Part model, mm, in its own coordinate system. Face numbers are marked on the shaded views. A direction names the side the tool comes from. Round coordinates to 2 decimals unless told otherwise and drop trailing zeros. Write each loop counter-clockwise with the first axis right and the second up, starting at its lowest first coordinate (ties: lowest second). Pieces come first, ordered by that corner, then holes.
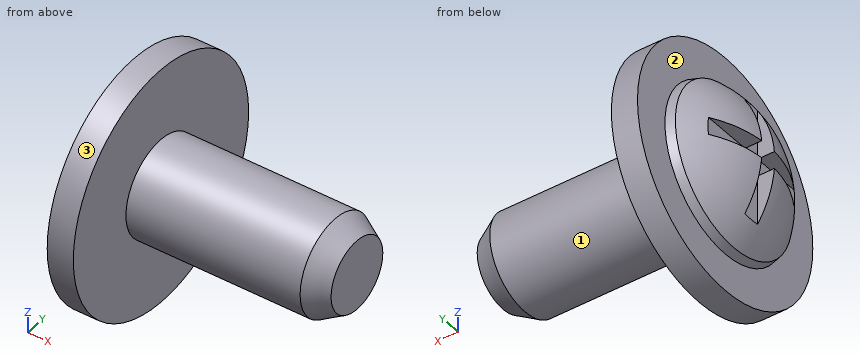
```python
from build123d import *

# Parameters (mm, degrees)
ESQUISSE2_W                  = 0.4
ESQUISSE2_H                  = 0.4
ENL_V_MAT_EXTRU_1_DEPTH      = 6.353036521
R_P_TITION_CIRCULAIRE1_COUNT = 2
R_P_TITION_CIRCULAIRE1_ANGLE = 90
ESQUISSE3_R                  = 2.75
BOSS_EXTRU_1_DEPTH           = 0.6


with BuildPart() as part:
    # Esquisse1 → Révolution1 (revolve)
    with BuildSketch(Plane.XY, mode=Mode.PRIVATE) as r_volution1_sk:
        with BuildLine():
            Line((0, 1.1), (0, 2.05))
            Line((0, 2.05), (-0.8, 1.835640646))
            ThreePointArc((-0.8, 1.835640646), (-1.391310546, 1.001196357), (-1.6, 0))
            Line((-1.6, 0), (4.5, 0))
            Line((4.5, 0), (4.5, 0.811324865))
            Line((4.5, 0.811324865), (4, 1.1))
            Line((4, 1.1), (0, 1.1))
        make_face()
    revolve(r_volution1_sk.sketch.rotate(Axis((-2.182265798, 0, 0), (1, 0, 0)), 90), axis=Axis((-2.182265798, 0, 0), (1, 0, 0)))

    # Esquisse2 → Enlèv. mat.-Extru.1 (cut, symmetric)
    with BuildSketch(Plane.XY):
        with Locations((-1.4, 0)):
            Rectangle(ESQUISSE2_W, ESQUISSE2_H)
    enl_v_mat_extru_1 = extrude(amount=ENL_V_MAT_EXTRU_1_DEPTH, both=True, mode=Mode.SUBTRACT)

    # Répétition circulaire1: Enlèv. mat.-Extru.1 ×2 about axis
    r_p_tition_circulaire1_axis = Axis((-2.182265798, 0, 0), (-1, 0, 0))
    for i in range(1, R_P_TITION_CIRCULAIRE1_COUNT):
        add(enl_v_mat_extru_1.rotate(r_p_tition_circulaire1_axis, i * R_P_TITION_CIRCULAIRE1_ANGLE / (R_P_TITION_CIRCULAIRE1_COUNT - 1)), mode=Mode.SUBTRACT)

    # Esquisse3 → Boss.-Extru.1 (add)
    with BuildSketch(Plane(origin=(0, 0, 0), x_dir=(0, 0, -1), z_dir=(1, 0, 0))):
        Circle(ESQUISSE3_R)
    extrude(amount=-BOSS_EXTRU_1_DEPTH)


solid = part.part
```
Q1. Which spindle directions (+Z, -Z, +X, -X, +Y, -Y) get a long thin tool onto all of the face, cutting with end or side? Do the marked faces 1, 2 and 3. Say none if no direction does.
Values follow:
face 1: +X
face 2: -X
face 3: +X, -X
Q2. Cut at D-D on y = 2. Write the cut outline in (x, z).
Values follow:
outline: (-0.6, -1.89) - (0, -1.89) - (0, 1.89) - (-0.6, 1.89) - close
Q3. Cut at C-C on x = 0.5. Write the cut outline in (y, z), plus the area to 3 significant figures.
Values follow:
outline: circle Ø2.2 at (0, 0)
area: 3.80 mm2
Q4. Drop flat-ended pins along their axis: pin 1 (1 mm diameter, centred on y = 1.5, z = 0, fed in from -X); pin 2 (2 mm diameter, centred on y = 2, z = 0, fed in from +X); pin 3 (3 mm diameter, centred on x = 2.5, z = 0.5, fed in from +Y). Give the stop position or say it passes through.
Values follow:
pin 1: stops at x = -1.36
pin 2: stops at x = 4.17
pin 3: stops at y = 1.1
Q5. Cut at A-A on y = 0. Write the cut outline in (x, z).
Values follow:
outline: (-1.2, -1.36) arc R2.51 ccw to (-0.8, -1.84) - (-0.6, -1.89) - (-0.6, -2.75) - (0, -2.75) - (0, -1.1) - (4, -1.1) - (4.5, -0.81) - (4.5, 0.81) - (4, 1.1) - (0, 1.1) - (0, 2.75) - (-0.6, 2.75) - (-0.6, 1.89) - (-0.8, 1.84) arc R2.51 ccw to (-1.2, 1.36) - close
Q6. Wall check: L1, parallel to X at y = -1.85, z = -1.6; L2, parallel to X at y = 0.25, z = -0.15; L3, parallel to Z at x = -0.25, y = -0.1. Give the ranges that are in metal, low to high.
Values follow:
L1: x = -0.6 to 0
L2: x = -1.2 to 4.5
L3: z = -2.75 to 2.75
